from build123d import *

# Parameters (mm, degrees)
SKETCH1_R                = 4
BOSS_EXTRUDE1_DEPTH      = 2.5
FILLET1_R                = 2
FILLET2_R                = 1
M4_CLEARANCE_HOLE1_D     = 4.5
M4_CLEARANCE_HOLE1_DEPTH = 5.2
M4_CLEARANCE_HOLE1_TIP   = 1.351936393


with BuildPart() as part:
    # Sketch1 → Boss-Extrude1 (new, symmetric)
    with BuildSketch(Plane(origin=(0, 0, 0), x_dir=(1, 0, 0), z_dir=(0, 1, 0))):
        with BuildLine():
            Line((95.549512883, 91.833784131), (91.833784131, 95.549512883))
            Line((91.833784131, 95.549512883), (79.549512883, 95.549512883))
            ThreePointArc((79.549512883, 95.549512883), (76.013978978, 94.085046789), (74.549512883, 90.549512883))
            Line((74.549512883, 90.549512883), (74.549512883, 88.691648507))
            Line((74.549512883, 88.691648507), (70.40737726, 84.549512883))
            Line((70.40737726, 84.549512883), (68.549512883, 84.549512883))
            ThreePointArc((68.549512883, 84.549512883), (65.013978978, 83.085046789), (63.549512883, 79.549512883))
            Line((63.549512883, 79.549512883), (63.549512883, 74.863221382))
            Line((63.549512883, 74.863221382), (43.937554159, 55.251262658))
            ThreePointArc((43.937554159, 55.251262658), (32.582736951, 47.664216362), (19.188816818, 45))
            Line((19.188816818, 45), (0, 45))
            Line((0, 45), (0, 37.5))
            Line((0, 37.5), (7.5, 37.5))
            Line((7.5, 37.5), (7.5, 30))
            Line((7.5, 30), (30, 30))
            Line((30, 30), (30, 7.5))
            Line((30, 7.5), (37.5, 7.5))
            Line((37.5, 7.5), (37.5, 0))
            Line((37.5, 0), (45, 0))
            Line((45, 0), (45, 19.188816818))
            ThreePointArc((45, 19.188816818), (47.664216362, 32.582736951), (55.251262658, 43.937554159))
            Line((55.251262658, 43.937554159), (74.863221382, 63.549512883))
            Line((74.863221382, 63.549512883), (79.549512883, 63.549512883))
            ThreePointArc((79.549512883, 63.549512883), (83.085046789, 65.013978978), (84.549512883, 68.549512883))
            Line((84.549512883, 68.549512883), (84.549512883, 70.40737726))
            Line((84.549512883, 70.40737726), (88.691648507, 74.549512883))
            Line((88.691648507, 74.549512883), (90.549512883, 74.549512883))
            ThreePointArc((90.549512883, 74.549512883), (94.085046789, 76.013978978), (95.549512883, 79.549512883))
            Line((95.549512883, 79.549512883), (95.549512883, 91.833784131))
        make_face()
        with Locations(Location((79.549512883, 79.549512883, 0), (0, 0, 270))):
            Circle(SKETCH1_R, mode=Mode.SUBTRACT)
        with BuildLine():
            Line((87.549512883, 81.249512883), (90.549512883, 81.249512883))
            ThreePointArc((90.549512883, 81.249512883), (92.249512883, 79.549512883), (90.549512883, 77.849512883))
            Line((90.549512883, 77.849512883), (87.549512883, 77.849512883))
            ThreePointArc((87.549512883, 77.849512883), (85.849512883, 79.549512883), (87.549512883, 81.249512883))
        make_face(mode=Mode.SUBTRACT)
        with BuildLine():
            Line((81.249512883, 71.549512883), (81.249512883, 68.549512883))
            ThreePointArc((81.249512883, 68.549512883), (79.549512883, 66.849512883), (77.849512883, 68.549512883))
            Line((77.849512883, 68.549512883), (77.849512883, 71.549512883))
            ThreePointArc((77.849512883, 71.549512883), (79.549512883, 73.249512883), (81.249512883, 71.549512883))
        make_face(mode=Mode.SUBTRACT)
        with BuildLine():
            Line((71.549512883, 77.849512883), (68.549512883, 77.849512883))
            ThreePointArc((68.549512883, 77.849512883), (66.849512883, 79.549512883), (68.549512883, 81.249512883))
            Line((68.549512883, 81.249512883), (71.549512883, 81.249512883))
            ThreePointArc((71.549512883, 81.249512883), (73.249512883, 79.549512883), (71.549512883, 77.849512883))
        make_face(mode=Mode.SUBTRACT)
        with BuildLine():
            Line((77.849512883, 87.549512883), (77.849512883, 90.549512883))
            ThreePointArc((77.849512883, 90.549512883), (79.549512883, 92.249512883), (81.249512883, 90.549512883))
            Line((81.249512883, 90.549512883), (81.249512883, 87.549512883))
            ThreePointArc((81.249512883, 87.549512883), (79.549512883, 85.849512883), (77.849512883, 87.549512883))
        make_face(mode=Mode.SUBTRACT)
    extrude(amount=BOSS_EXTRUDE1_DEPTH, both=True)

    # Fillet1
    fillet1_edges = [part.edges().sort_by_distance(p)[0] for p in [
        (91.833784131, 0, -95.549512883),
        (95.549512883, 0, -91.833784131),
        (88.691648507, 0, -74.549512883),
        (84.549512883, 0, -70.40737726),
        (74.863221382, 0, -63.549512883),
        (30, 0, -30),
        (63.549512883, 0, -74.863221382),
        (70.40737726, 0, -84.549512883),
        (74.549512883, 0, -88.691648507),
    ]]
    fillet(fillet1_edges, radius=FILLET1_R)

    # Fillet2
    fillet2_edges = [part.edges().sort_by_distance(p)[0] for p in [
        (45, 0, 0),
        (37.5, 0, 0),
        (37.5, 0, -7.5),
        (30, 0, -7.5),
        (7.5, 0, -30),
        (7.5, 0, -37.5),
        (0, 0, -37.5),
        (0, 0, -45),
    ]]
    fillet(fillet2_edges, radius=FILLET2_R)

    # M4 Clearance Hole1
    with Locations(Plane(origin=(0, 2.5, 0), x_dir=(1, 0, 0), z_dir=(0, 1, 0))):
        with Locations((15, 37.5), (37.5, 15), (37.5, 37.5)):
            Hole(M4_CLEARANCE_HOLE1_D / 2, depth=M4_CLEARANCE_HOLE1_DEPTH)
            with Locations((0, 0, -(M4_CLEARANCE_HOLE1_DEPTH + M4_CLEARANCE_HOLE1_TIP / 2))):  # 118° drill point
                Cone(0, M4_CLEARANCE_HOLE1_D / 2, M4_CLEARANCE_HOLE1_TIP, mode=Mode.SUBTRACT)


solid = part.part
Read the model definition and answer for the solid it produces. Units are mm, in the model's axes. A direction names the side the tool comes from. Give positions to 0.01 mm unless a question says otherwise; leave off trailing zeros. Write each loop counter-clockwise with the first axis right and the second up, starting at its lowest first coordinate (ties: lowest second). Pieces come first, ordered by that corner, then holes. Notation, with made-up numbers: (16, 48.25) - (30, 48.25) arc R29 cw to (30, 69.25) - close; hole circle Ø7 at (38.25, -17.5). An arc over 180 degrees is marked (long way). Use CSV: the item, a comma, the result in double quotes. Start each with the question number.
Item 1: The part is cut by section A-A, the plane x = 15. Give the vertices of the cut face in (y, z).
Item 2: Flat-ended cylindrical pins translate along their axes: P1, Ø3, axis at x = 59, y = 1, coming from the -Z side; P2, Ø2.5, axis at x = 89, y = -1, coming from the +Z side; P3, Ø2.5, axis at y = 0, z = -5, coming from the -X side. Find the tip coordinate at first contact, or state that the pin passes through.
Item 3: The part is cut by section B-B, the plane z = -15. Give the vertices of the cut face in (x, y), and give its area (3 significant figures).
Item 4: For faces 1 (the flat face through (10, 0, -45)), 2 (the flat face through (18, 0, -30)), 3 (the flat face through (78, 0, -63.55)), 4 (the flat face through (70, 0, -81.25)), determine the directions among +Z, -Z, +X, -X, +Y, -Y from which every point of the face is accessible in a straight line to the end or side of a thin tool.
Item 5: The part is cut by section C-C, the plane y = -0.6. Count the separate pieces of the cut face and the enclosed holes in it, and give its area (3 significant figures).
Item 6: The part is cut by section D-D, the plane x = 33. Give the vertices of the cut face in (y, z), and give its area (3 significant figures).
Item 7: Consider line 1 (Z direction, x = 15, y = 0.25); line 2 (X direction, y = 0.9, z = -19); line 3 (Z direction, x = 81, y = -0.6). Determine where each line is inside the solid, lowest interval first.
Item 8: The mould has two halves that part along Z. Classify faces 5 (the flat face through (64.631, 0.035, -53.317)), 6 (the cylindrical face through (79.51, 0.04, -92.25)), 7 (the flat face through (53.584, 0.035, -64.898)), 8 (the flat face through (37.5, 0, -4)): pulls with the +Z half, pulls with the -Z half, needs draft (parallel to the pull), parting line crosses it, or undercut.
Taken from the geometry:
1,outline,"(-2.5, -45) - (2.5, -45) - (2.5, -39.75) - (-2.5, -39.75) - close; (-2.5, -35.25) - (2.5, -35.25) - (2.5, -30) - (-2.5, -30) - close"
2,P1,"z = -71.81"
2,P2,"z = -73.61"
2,P3,"x = 37.5"
3,outline,"(30, -2.5) - (35.25, -2.5) - (35.25, 2.5) - (30, 2.5) - close; (39.75, -2.5) - (45, -2.5) - (45, 2.5) - (39.75, 2.5) - close"
3,area,"52.5 mm2"
4,face 1,"-Z, -X, +Y, -Y"
4,face 2,"+Z, -X, +Y, -Y"
4,face 3,"+Z, +X, +Y, -Y"
4,face 4,"+Y, -Y"
5,separate pieces,"1"
5,enclosed holes,"8"
5,area,"2,210 mm2"
6,outline,"(-2.5, -47.84) - (2.5, -47.84) - (2.5, -7.5) - (-2.5, -7.5) - close"
6,area,"202 mm2"
7,line 1,"-45 to -39.75, -35.25 to -30"
7,line 2,"30 to 45"
7,line 3,"-95.55 to -91.44, -86.66 to -83.28, -75.82 to -72.44, -67.66 to -63.76"
8,face 5,"pulls with the +Z half"
8,face 6,"undercut"
8,face 7,"pulls with the -Z half"
8,face 8,"needs draft"
